```python
from build123d import *

# Parameters (mm, degrees)
SKETCH1_R           = 1.5
SKETCH1_R_2         = 4.000000004
SKETCH1_W           = 15.264959334
SKETCH1_H           = 28.225795916
SKETCH1_W_2         = 16.875415015
SKETCH1_H_2         = 37.724658957
BOSS_EXTRUDE1_DEPTH = 4


with BuildPart() as part:
    # Sketch1 → Boss-Extrude1 (new body)
    with BuildSketch(Plane.XY):
        with BuildLine():
            Line((-30.000000002, 34.937585276), (-30.000000002, -5e-09))
            Line((-30.000000002, -5e-09), (-18.500000007, -5e-09))
            ThreePointArc((-18.500000007, -5e-09), (-18.398655071, -1.933776576), (-18.09573062, -3.846366286))
            Line((-18.09573062, -3.846366286), (-29.344428024, -6.23735073))
            ThreePointArc((-29.344428024, -6.23735073), (-28.53169549, -9.270509837), (-27.406363731, -12.202099298))
            Line((-27.406363731, -12.202099298), (-16.900590972, -7.524627904))
            ThreePointArc((-16.900590972, -7.524627904), (-16.021469975, -9.250000008), (-14.966814401, -10.874027176))
            Line((-14.966814401, -10.874027176), (-24.270509832, -17.633557574))
            ThreePointArc((-24.270509832, -17.633557574), (-22.294344765, -20.073918196), (-20.073918191, -22.294344769))
            Line((-20.073918191, -22.294344769), (-12.378916221, -13.74817928))
            ThreePointArc((-12.378916221, -13.74817928), (-10.87402717, -14.966814404), (-9.250000002, -16.021469978))
            Line((-9.250000002, -16.021469978), (-14.999999999, -25.980762117))
            ThreePointArc((-14.999999999, -25.980762117), (-12.202099292, -27.406363733), (-9.27050983, -28.531695491))
            Line((-9.27050983, -28.531695491), (-5.716814397, -17.594545559))
            ThreePointArc((-5.716814397, -17.594545559), (-3.846366281, -18.09573062), (-1.933776571, -18.39865507))
            Line((-1.933776571, -18.39865507), (-3.135853898, -29.835656862))
            ThreePointArc((-3.135853898, -29.835656862), (0, -30.000000001), (3.135853897, -29.835656861))
            Line((3.135853897, -29.835656861), (1.93377657, -18.398655069))
            ThreePointArc((1.93377657, -18.398655069), (3.84636628, -18.095730618), (5.716814395, -17.594545555))
            Line((5.716814395, -17.594545555), (9.270509829, -28.531695488))
            ThreePointArc((9.270509829, -28.531695488), (12.202099289, -27.406363728), (14.999999996, -25.980762112))
            Line((14.999999996, -25.980762112), (9.249999999, -16.021469973))
            ThreePointArc((9.249999999, -16.021469973), (10.874027165, -14.966814398), (12.378916215, -13.748179274))
            Line((12.378916215, -13.748179274), (20.073918185, -22.294344763))
            ThreePointArc((20.073918185, -22.294344763), (22.294344757, -20.07391819), (24.270509823, -17.633557568))
            Line((24.270509823, -17.633557568), (14.966814392, -10.87402717))
            ThreePointArc((14.966814392, -10.87402717), (16.021469966, -9.250000002), (16.900590962, -7.5246279))
            Line((16.900590962, -7.5246279), (27.40636372, -12.202099293))
            ThreePointArc((27.40636372, -12.202099293), (28.531695479, -9.270509833), (29.344428012, -6.237350727))
            Line((29.344428012, -6.237350727), (18.095730608, -3.846366284))
            ThreePointArc((18.095730608, -3.846366284), (18.398655059, -1.933776575), (18.499999994, -5e-09))
            Line((18.499999994, -5e-09), (29.999999989, -5e-09))
            Line((29.999999989, -5e-09), (29.999999989, 34.937585276))
            Line((29.999999989, 34.937585276), (25.999999989, 34.935484549))
            Line((25.999999989, 34.935484549), (25.999999989, 54.935484549))
            Line((25.999999989, 54.935484549), (29.999999989, 54.937585276))
            Line((29.999999989, 54.937585276), (29.999999989, 94.937585276))
            Line((29.999999989, 94.937585276), (25.999999989, 94.935484549))
            Line((25.999999989, 94.935484549), (25.999999989, 114.935484549))
            Line((25.999999989, 114.935484549), (29.999999989, 114.937585276))
            Line((29.999999989, 114.937585276), (29.999999989, 154.937585276))
            Line((29.999999989, 154.937585276), (25.999999989, 154.935484549))
            Line((25.999999989, 154.935484549), (25.999999989, 174.935484549))
            Line((25.999999989, 174.935484549), (29.999999989, 174.937585276))
            Line((29.999999989, 174.937585276), (29.999999989, 214.937585276))
            Line((29.999999989, 214.937585276), (25.999999989, 214.935484549))
            Line((25.999999989, 214.935484549), (25.999999989, 234.935484549))
            Line((25.999999989, 234.935484549), (29.999999989, 234.937585276))
            Line((29.999999989, 234.937585276), (29.999999989, 317.280454814))
            Line((29.999999989, 317.280454814), (-30.000000002, 317.280454814))
            Line((-30.000000002, 317.280454814), (-30.000000002, 234.937585276))
            Line((-30.000000002, 234.937585276), (-26.000000002, 234.935484549))
            Line((-26.000000002, 234.935484549), (-26.000000002, 214.935484549))
            Line((-26.000000002, 214.935484549), (-30.000000002, 214.937585276))
            Line((-30.000000002, 214.937585276), (-30.000000002, 174.937585276))
            Line((-30.000000002, 174.937585276), (-26.000000002, 174.935484549))
            Line((-26.000000002, 174.935484549), (-26.000000002, 154.935484549))
            Line((-26.000000002, 154.935484549), (-30.000000002, 154.937585276))
            Line((-30.000000002, 154.937585276), (-30.000000002, 114.937585276))
            Line((-30.000000002, 114.937585276), (-26.000000002, 114.935484549))
            Line((-26.000000002, 114.935484549), (-26.000000002, 94.935484549))
            Line((-26.000000002, 94.935484549), (-30.000000002, 94.937585276))
            Line((-30.000000002, 94.937585276), (-30.000000002, 54.937585276))
            Line((-30.000000002, 54.937585276), (-26.000000002, 54.935484549))
            Line((-26.000000002, 54.935484549), (-26.000000002, 34.935484549))
            Line((-26.000000002, 34.935484549), (-30.000000002, 34.937585276))
        make_face()
        with Locations((14.272904266, 226.626719069)):
            Circle(SKETCH1_R, mode=Mode.SUBTRACT)
        with Locations((-6e-09, -5e-09)):
            Circle(SKETCH1_R_2, mode=Mode.SUBTRACT)
        with Locations((14.272904266, 181.743471482)):
            Circle(SKETCH1_R, mode=Mode.SUBTRACT)
        with Locations((-16.500000002, 148.89892656)):
            Circle(SKETCH1_R, mode=Mode.SUBTRACT)
        with Locations((-16.500000002, 109.235963146)):
            Circle(SKETCH1_R, mode=Mode.SUBTRACT)
        with Locations((14.272904266, 80.661965148)):
            Circle(SKETCH1_R, mode=Mode.SUBTRACT)
        with Locations((14.272904266, 43.392817658)):
            Circle(SKETCH1_R, mode=Mode.SUBTRACT)
        Polygon((-11.924742875, 260.626143035), (0, 260.626143035), (-2e-09, 234.935484549), (-11.924742875, 234.935484549), align=None, mode=Mode.SUBTRACT)
        with Locations((7.963115832, 134.786028602)):
            Rectangle(SKETCH1_W, SKETCH1_H, mode=Mode.SUBTRACT)
        with Locations((-4.43770751, 48.307901023)):
            Rectangle(SKETCH1_W_2, SKETCH1_H_2, mode=Mode.SUBTRACT)
    extrude(amount=BOSS_EXTRUDE1_DEPTH)


solid = part.part
```
Model file for the job. Use its own axes, mm. A direction names the side the tool comes from. Coordinates: 2 decimals unless noted, no trailing zeros. Order: outer loops, then holes, each group sorted by start corner. A loop starts at its lowest first (then second) coordinate and runs counter-clockwise, first axis right, second up. Notation, with made-up numbers: (34, 68.5) -> (92, 68.5) arc R25 ccw to (92, 90.5) -> close; hole circle Ø9 at (-9, 4). An arc over 180 degrees is marked (long way). Answer as a JSON object with one key per item and string values. Group by question number.
1) Which spindle directions (+Z, -Z, +X, -X, +Y, -Y) get a long thin tool onto all of the face, cutting with end or side? Do faces 1 (the face through (-19.554, -14.206, 1.972)), 2 (the face through (0, 146, 0)). Say none if no direction does.
2) Flat gauge pins, fed straight in: pin 1 (2 mm diameter, centred on y = 161, z = 1.5, fed in from +X); pin 2 (5 mm diameter, centred on x = -0.5, y = 43.5, fed in from -Z); pin 3 (3 mm diameter, centred on x = 17, y = 246.5, fed in from -Z); pin 4 (2 mm diameter, centred on y = 169, z = 3, fed in from -X). Where does each tip first touch, or does it go through?
3) Drill centre lines: L1, parallel to Y at x = -16.5, z = 2.8; L2, parallel to Y at x = -11.5, z = 2.9; L3, parallel to Y at x = 21, z = 2.6. Where is each one in solid material? Low to high.
4) Pull direction Y, two halves, no side cores. Call faces 3 (the face through (12.165, -21.071, 1.972)), 4 (the face through (0, 146, 4)): +Y half, -Y half, draft (parallel to the pull), parting line (faces both ways), or undercut.
5) Cut at A-A, the plane y = 257. Write the cut outline in (x, z), then the cut area to 3 significant figures.
6) Cut at B-B, the plane z = 2.9. Count the separate pieces of the cut face and the enclosed holes in it, then the cut area to 3 significant figures.
Check values:
{
 "1": {"face 1": "+Z, -Z", "face 2": "-Z, +X, -X, +Y, -Y"},
 "2": {"pin 1": "stops at x = 26", "pin 2": "passes through", "pin 3": "stops at z = 0", "pin 4": "stops at x = -26"},
 "3": {"L1": "y = -18.33 to -11.99, -8.37 to 107.74, 110.74 to 147.4, 150.4 to 317.28", "L2": "y = -27.71 to -19.92, -14.49 to 29.45, 67.17 to 234.94, 260.63 to 317.28", "L3": "y = -21.42 to -15.26, -9.35 to -4.46, 0 to 317.28"},
 "4": {"face 3": "undercut", "face 4": "draft"},
 "5": {"outline": "(-30, 0) -> (-11.92, 0) -> (-11.92, 4) -> (-30, 4) -> close; (0, 0) -> (30, 0) -> (30, 4) -> (0, 4) -> close", "area": "192 mm²"},
 "6": {"separate pieces": "1", "enclosed holes": "10", "area": "17,900 mm²"}
}
